The model under review builds one solid part; all positions refer to its coordinate system, in mm. Face numbers are marked on the shaded views. A direction names the side the tool comes from. Coordinates: 2 decimals unless noted, no trailing zeros. Loops run counter-clockwise (first coordinate to the right, second up) from the corner with the lowest first, then second, coordinate; pieces in that order, holes last. Notation, with made-up numbers: (86.25, 87) - (127.25, 87) arc R22 cw to (127.25, 111) - close; hole circle Ø5 at (81.25, -12). An arc over 180 degrees is marked (long way). One line per item, written item: value. Start each with the question number.
1. We need section B-B, the plane y = 0. Give the boundary of the cut face in (x, z).
2. We need section D-D, the plane y = 8. Give the boundary of the cut face in (x, z), then the cut area to 3 significant figures.
3. We need section A-A, the plane x = -15.5. Give the boundary of the cut face in (y, z), then the cut area to 3 significant figures.
4. For the marked faces 1 and 2, list the 3-axis set-ups (+Z, -Z, +X, -X, +Y, -Y) from which the entire face can be reached by the end or side of a thin tool; tool diameter is ignored.
5. To check wall thickness, follow line 1 (Y direction, x = -17.5, z = 27.5); line 2 (X direction, y = 0.5, z = 66.5); line 3 (Z direction, x = 0, y = -11.55). State the ranges of each line that lie inside material, in increasing order.
6. We need section C-C, the plane z = 19. Give the boundary of the cut face in (x, y), then the cut area to 3 significant figures.
7. Mouldability with a two-part tool opening along Y and no side actions: class the marked faces 3, 4 and 5 as +Y half, -Y half, draft (parallel to the pull), parting line (faces both ways), or undercut.
from build123d import *

# Parameters (mm, degrees)
SKETCH1_W               = 50.8
SKETCH1_H               = 25.4
SKETCH1_W_2             = 47.625
SKETCH1_H_2             = 22.225
BOSS_EXTRUDE1_DEPTH     = 101.6
SKETCH2_R               = 14.2875
CUT_EXTRUDE1_DEPTH      = 26.4
SKETCH3_R               = 3.6195
CUT_EXTRUDE2_DEPTH      = 1
CUT_EXTRUDE2_DEPTH_BACK = 51.8


with BuildPart() as part:
    # Sketch1 → Boss-Extrude1 (new body)
    with BuildSketch(Plane.XY):
        Rectangle(SKETCH1_W, SKETCH1_H)
        Rectangle(SKETCH1_W_2, SKETCH1_H_2, mode=Mode.SUBTRACT)
    extrude(amount=BOSS_EXTRUDE1_DEPTH)

    # Sketch2 → Cut-Extrude1 (cut, through all)
    with BuildSketch(Plane.XZ.offset(12.7)):
        with Locations((0, 76.2)):
            Circle(SKETCH2_R)
    extrude(amount=-CUT_EXTRUDE1_DEPTH, mode=Mode.SUBTRACT)

    # Sketch3 → Cut-Extrude2 (cut, two sides)
    with BuildSketch(Plane(origin=(25.4, 0, 0), x_dir=(0, 0, -1), z_dir=(1, 0, 0))) as cut_extrude2_sk:
        with Locations((-38.1381, 0)):
            Circle(SKETCH3_R)
        with Locations((-12.6365, 0)):
            Circle(SKETCH3_R)
    extrude(amount=CUT_EXTRUDE2_DEPTH, mode=Mode.SUBTRACT)
    extrude(cut_extrude2_sk.sketch, amount=-CUT_EXTRUDE2_DEPTH_BACK, mode=Mode.SUBTRACT)


solid = part.part
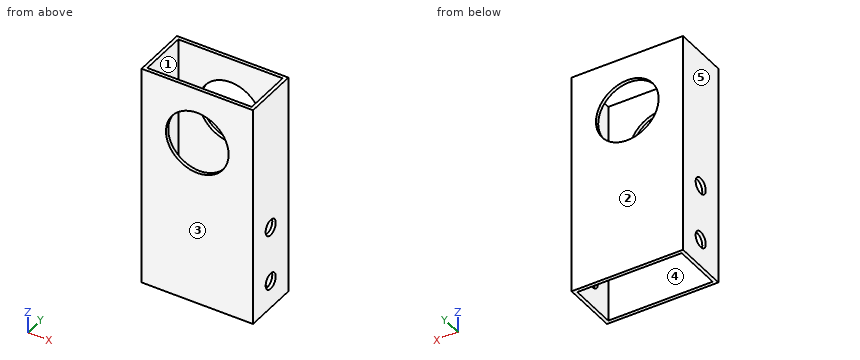
Findings below:
1. outline: (-25.4, 0) - (-23.81, 0) - (-23.81, 9.02) - (-25.4, 9.02) - close; (-25.4, 16.26) - (-23.81, 16.26) - (-23.81, 34.52) - (-25.4, 34.52) - close; (-25.4, 41.76) - (-23.81, 41.76) - (-23.81, 101.6) - (-25.4, 101.6) - close; (23.81, 0) - (25.4, 0) - (25.4, 9.02) - (23.81, 9.02) - close; (23.81, 16.26) - (25.4, 16.26) - (25.4, 34.52) - (23.81, 34.52) - close; (23.81, 41.76) - (25.4, 41.76) - (25.4, 101.6) - (23.81, 101.6) - close
2. outline: (-25.4, 0) - (-23.81, 0) - (-23.81, 101.6) - (-25.4, 101.6) - close; (23.81, 0) - (25.4, 0) - (25.4, 101.6) - (23.81, 101.6) - close
2. area: 323 mm2
3. outline: (-12.7, 0) - (-11.11, 0) - (-11.11, 101.6) - (-12.7, 101.6) - close; (11.11, 0) - (12.7, 0) - (12.7, 101.6) - (11.11, 101.6) - close
3. area: 323 mm2
4. face 1: +Z, -Z
4. face 2: +Z, -Z, +X, -X, +Y
5. line 1: -12.7 to -11.11, 11.11 to 12.7
5. line 2: -25.4 to -23.81, 23.81 to 25.4
5. line 3: 0 to 61.91, 90.49 to 101.6
6. outline: (-25.4, -12.7) - (25.4, -12.7) - (25.4, 12.7) - (-25.4, 12.7) - close; hole (-23.81, -11.11) - (23.81, -11.11) - (23.81, 11.11) - (-23.81, 11.11) - close
6. area: 232 mm2
7. face 3: -Y half
7. face 4: undercut
7. face 5: draft
